Autodesk Inventor part; units mm, degrees
ref_plane "YZ Plane" through (0, 0, 0) normal (1, 0, 0) x (0, 1, 0)
ref_plane "XZ Plane" through (0, 0, 0) normal (0, 1, 0) x (-1, 0, 0)
ref_plane "XY Plane" through (0, 0, 0) normal (0, 0, 1) x (1, 0, 0)
sketch "Sketch1" plane through (0, 0, 0) normal (0, 0, 1) x (1, 0, 0)
  line L0 (-74.8322, 32.4161) -> (-4.8322, 32.4161)
  line L1 (5.1678, 22.4161) -> (5.1678, -47.5839)
  line L2 (-4.8322, -57.5839) -> (-74.8322, -57.5839)
  line L3 (-84.8322, -47.5839) -> (-84.8322, 22.4161)
  arc A0 (-74.8322, 32.4161) -> (-84.8322, 22.4161) centre (-74.8322, 22.4161) ccw
  arc A1 (5.1678, 22.4161) -> (-4.8322, 32.4161) centre (-4.8322, 22.4161) ccw
  arc A2 (-4.8322, -57.5839) -> (5.1678, -47.5839) centre (-4.8322, -47.5839) ccw
  arc A3 (-84.8322, -47.5839) -> (-74.8322, -57.5839) centre (-74.8322, -47.5839) ccw
  point P0 (0, 0)
  point P1 (-84.8322, 32.4161)
  point P2 (5.1678, 32.4161)
  point P3 (-84.8322, -57.5839)
  dimension "d0" = 90
  dimension "d1" = 90
  dimension "d2" = 10
extrude "Extrusion1" add sketch "Sketch1" along normal blind 6
sketch "Sketch2" plane through (0, 0, 6) normal (0, 0, 1) x (1, 0, 0)
  line L0 (-84.8322, -47.5839) -> (-84.8322, 22.4161)
  line L1 (-84.8322, -12.5839) -> (5.1678, -12.5839) construction
  line L2 (5.1678, 22.4161) -> (5.1678, -47.5839)
  circle A0 centre (-39.8322, -12.5839) radius 30.5
  point P0 (0, 0)
  dimension "d5" = 61
extrude "Extrusion2" cut sketch "Sketch2" against normal through all
sketch "Sketch3" plane through (0, 0, 6) normal (0, 0, 1) x (1, 0, 0)
  line L0 (5.1678, -47.5839) -> (5.1678, 22.4161)
  line L1 (5.1678, -12.5839) -> (30.1678, -12.5839) construction
  line L2 (26.381, -52.2971) -> (5.1678, -31.0839)
  circle A0 centre (-39.8322, -12.5839) radius 30.5
  line L3 (-39.8322, -12.5839) -> (-18.2655, 8.9829) construction
  line L4 (-79.5454, 53.6293) -> (-58.3322, 32.4161)
  line L5 (-74.8322, -57.5839) -> (-4.8322, -57.5839)
  line L6 (-4.8322, -57.5839) -> (31.1678, -57.5839)
  line L7 (31.1678, -57.5839) -> (26.381, -52.2971)
  arc A1 (-74.8322, 32.4161) -> (-84.8322, 22.4161) centre (-74.8322, 22.4161) ccw
  line L8 (-84.8322, 22.4161) -> (-84.8322, 58.9161)
  line L9 (-84.8322, 58.9161) -> (-79.5454, 53.6293)
  line L10 (-4.8322, 32.4161) -> (-74.8322, 32.4161)
  line L11 (-58.3322, 32.4161) -> (-74.8322, 32.4161)
  arc A2 (-4.8322, -57.5839) -> (5.1678, -47.5839) centre (-4.8322, -47.5839) ccw
  line L12 (5.1678, -31.0839) -> (5.1678, -47.5839)
  point P0 (0, 0)
  dimension "d13" = 53.5
extrude "Extrusion3" add sketch "Sketch3" against normal up to surface (6 mm away) contours L0 L2 L7 L6 A2 | L4 L10 A1 L8 L9
fillet "Fillet1" radius 7 2 edges at (-58.3322, 32.4161, 3) (5.1678, -31.0839, 3)
sketch "Sketch4" plane through (0, 0, 0) normal (0, 0, -1) x (-1, 0, 0)
  circle A0 centre (74.6322, 22.2161) radius 3.25
  circle A1 centre (74.6322, -47.3839) radius 3.25
  circle A2 centre (5.0322, -47.3839) radius 3.25
  circle A3 centre (5.0322, 22.2161) radius 3.25
  point P0 (0, 0)
extrude "Extrusion4" cut sketch "Sketch4" against normal through all
properties part number "Motor support"
Source: CAD feature listing. Evaluate the final solid. Frame: model axes, mm. A direction names the side the tool comes from. Give positions to 0.01 mm unless a question says otherwise; leave off trailing zeros. Order: outer loops, then holes, each group sorted by start corner. A loop starts at its lowest first (then second) coordinate and runs counter-clockwise, first axis right, second up. Notation, with made-up numbers: (-22, -8) -> (34, -8) arc R12 ccw to (34, -1) -> close; hole circle Ø10 at (-27.75, 31.25). An arc over 180 degrees is marked (long way). Use a Markdown table: item, result.
1) Reachability of faces 1 (the cylindrical face through (-10.74, -3.42, 3.04)), 2 (the flat face through (5.168, -3, 3)) from +Z, -Z, +X, -X, +Y, -Y: full face, straight path, thin tool, end or side. Return the list, or none.
Answer list:
| item | result |
|---|---|
| face 1 | +Z, -Z |
| face 2 | +Z, -Z, +X, +Y |
2) Section query A-A, the plane x = -38. Return the cut outline in (y, z).
Answer list:
| item | result |
|---|---|
| outline | (-57.58, 0) -> (-43.03, 0) -> (-43.03, 6) -> (-57.58, 6) -> close; (17.86, 0) -> (32.42, 0) -> (32.42, 6) -> (17.86, 6) -> close |
3) Ray query, line 1 along Y through (x, z) = (-40.5, 2.35); line 2 along Y through (x, z) = (-6.5, 4.3); line 3 along X through (y, z) = (24, 4.35). Return the intervals inside material, ascending. Write a range as [from, to].
Answer list:
| item | result |
|---|---|
| line 1 | [-57.58, -43.08], [17.91, 32.42] |
| line 2 | [-57.58, -50.28], [-44.48, 19.32], [25.12, 32.42] |
| line 3 | [-84.83, -77.35], [-71.92, -7.75], [-2.32, 5.04] |
4) Section query B-B, the plane y = 2. Return the cut outline in (x, z).
Answer list:
| item | result |
|---|---|
| outline | (-84.83, 0) -> (-66.62, 0) -> (-66.62, 6) -> (-84.83, 6) -> close; (-13.04, 0) -> (5.17, 0) -> (5.17, 6) -> (-13.04, 6) -> close |
5) Mould query, pull axis Y, two halves, no side actions, for faces 3 (the cylindrical face through (-71.385, 22.359, 2.958)), 4 (the cylindrical face through (5.715, -30.899, 2.958)), 5 (the cylindrical face through (-81.83, -54.73, 2.96)). Classes: +Y half, -Y half, draft (parallel to the pull), parting line (faces both ways), or undercut.
Answer list:
| item | result |
|---|---|
| face 3 | undercut |
| face 4 | +Y half |
| face 5 | -Y half |
6) Section query D-D, the plane y = 46. Return the cut outline in (x, z).
Answer list:
| item | result |
|---|---|
| outline | (-84.83, 0) -> (-71.92, 0) -> (-71.92, 6) -> (-84.83, 6) -> close |
7) Section query C-C, the plane z = 3.75. Return the cut outline in (x, y), then the cut area to 3 significant figures.
Answer list:
| item | result |
|---|---|
| outline | (-84.83, -47.58) arc R10 ccw to (-74.83, -57.58) -> (31.17, -57.58) -> (26.38, -52.3) -> (7.22, -33.13) arc R7 cw to (5.17, -28.18) -> (5.17, 22.42) arc R10 ccw to (-4.83, 32.42) -> (-55.43, 32.42) arc R7 cw to (-60.38, 34.47) -> (-84.83, 58.92) -> close; hole circle Ø6.5 at (-74.63, -47.38); hole circle Ø6.5 at (-74.63, 22.22); hole circle Ø61 at (-39.83, -12.58); hole circle Ø6.5 at (-5.03, -47.38); hole circle Ø6.5 at (-5.03, 22.22) |
| area | 5,700 mm² |
8) Contact query for flat-ended pins moving along their axis: P1, Ø5, axis at x = -74.63, y = 22.22, coming from the -Z side; P2, Ø8.5, axis at x = -5.03, y = -47.38, coming from the +Z side; P3, Ø3, axis at x = -71.5, z = 1.5, coming from the +Y side; P4, Ø1.8, axis at x = -29.5, z = 1.5, coming from the +Y side. Output: stop coordinate, or through.
Answer list:
| item | result |
|---|---|
| P1 | through |
| P2 | z = 6 |
| P3 | y = 47.08 |
| P4 | y = 32.42 |
